from build123d import *

# Parameters (mm, degrees)
SKETCH1_W                   = 50.8
SKETCH1_H                   = 31.75
BASE_LEG_DEPTH              = 4.7625
SKETCH2_W                   = 50.8
SKETCH2_H                   = 31.75
PERPENDICULAR_LEG_DEPTH     = 4.7625
FILLET1_R                   = 2.032
F_32_0_116_DIAMETER_HOLE1_D = 2.9464
W_0_386_DIAMETER_HOLE1_D    = 9.8044
SKETCH15_W                  = 6.549717957
SKETCH15_H                  = 10.713777056
CUT_EXTRUDE2_DEPTH          = 3.81


with BuildPart() as part:
    # Sketch1 → Base leg (new body)
    with BuildSketch(Plane(origin=(0, 0, 0), x_dir=(1, 0, 0), z_dir=(0, 1, 0))):
        with Locations((25.4, -15.875)):
            Rectangle(SKETCH1_W, SKETCH1_H)
    extrude(amount=BASE_LEG_DEPTH)

    # Sketch2 → Perpendicular leg (add)
    with BuildSketch(Plane.XY):
        with Locations((25.4, 15.875)):
            Rectangle(SKETCH2_W, SKETCH2_H)
    extrude(amount=PERPENDICULAR_LEG_DEPTH)

    # Fillet1
    fillet1_edges = [part.edges().sort_by_distance(p)[0] for p in [
        (25.4, 31.75, 4.7625),
        (25.4, 4.7625, 31.75),
    ]]
    fillet(fillet1_edges, radius=FILLET1_R)

    # #32 (0.116) Diameter Hole1 (through all)
    with Locations(Plane(origin=(0, 0, 0), x_dir=(-1, 0, 0), z_dir=(0, -1, 0))):
        with Locations((-38.1, -19.05), (-12.7, -19.05)):
            Hole(F_32_0_116_DIAMETER_HOLE1_D / 2)

    # W (0.386) Diameter Hole1 (through all)
    with Locations(Plane(origin=(0, 0, 0), x_dir=(-1, 0, 0), z_dir=(0, 0, -1))):
        with Locations((-12.7, 19.05), (-38.1, 19.05)):
            Hole(W_0_386_DIAMETER_HOLE1_D / 2)

    # Sketch15 → Cut-Extrude2 (cut)
    with BuildSketch(Plane(origin=(0, 4.7625, 0), x_dir=(1, 0, 0), z_dir=(0, 1, 0))):
        with Locations((2.926349869, -25.756092966)):
            Rectangle(SKETCH15_W, SKETCH15_H)
    extrude(amount=-CUT_EXTRUDE2_DEPTH, mode=Mode.SUBTRACT)


solid = part.part
Input: part model. Units: mm. Frame: model coordinates. A direction names the side the tool comes from. Coordinates: 2 decimals unless noted, no trailing zeros. Loops run counter-clockwise (first coordinate to the right, second up) from the corner with the lowest first, then second, coordinate; pieces in that order, holes last. Notation, with made-up numbers: (84, -35) - (111, -35) arc R20 cw to (111, -30) - close; hole circle Ø1 at (80, -39.75). An arc over 180 degrees is marked (long way). Answer in a Markdown table with one row per item. Add a question column.
Item 1: Access query for faces 5 (the flat face through (0, 10, 4)), 6 (the flat face through (3, 3, 20.399)), 7 (the flat face through (25, 4.762, 17)). Directions: +Z, -Z, +X, -X, +Y, -Y. A direction counts if a zero-diameter tool reaches every point of the face in a straight line with its end or side. Return the directions, or none.
Item 2: Mould query, pull axis Z, two halves, no side actions, for faces 1 (the flat face through (6.201, 3, 26)), 2 (the flat face through (25, 16, 0)), 3 (the cylindrical face through (42.776, 20.522, 2.415)), 4 (the flat face through (25, 1, 31.75)). Classes: released by +Z, released by -Z, zero draft, split by the parting line, or undercut.
Item 3: Section query A-A on y = 19.05. Return the cut outline in (x, z).
Item 4: Contact query for flat-ended pins moving along their axis: P1, Ø5, axis at x = 10.5, z = 26, coming from the +Y side; P2, Ø5, axis at y = 8.5, z = 16, coming from the -X side; P3, Ø12.5, axis at x = 21.5, y = 22, coming from the +Z side; P4, Ø4, axis at x = 26, y = 19.5, coming from the -Z side. Output: stop coordinate, or through.
Item 5: Section query C-C on z = 19.05. Return the cut outline in (x, y).
Item 6: Section query D-D on y = 13.5. Return the cut outline in (x, z), then the cut area to 3 significant figures.
Item 7: Section query B-B on x = 12.7. Return the cut outline in (y, z).
Item 8: Line query: line 1 along X through (y, z) = (1.2, 19.05); line 2 along X through (y, z) = (19, 2); line 3 along Z through (x, y) = (38, 2). Output: solid intervals per line, ascending. Write a range as [from, to].
Recorded:
| question | item | result |
|---|---|---|
| 1 | face 5 | +Z, -Z, -X, +Y, -Y |
| 1 | face 6 | -X, +Y |
| 1 | face 7 | +Z, +X, -X, +Y |
| 2 | face 1 | undercut |
| 2 | face 2 | released by -Z |
| 2 | face 3 | zero draft |
| 2 | face 4 | released by +Z |
| 3 | outline | (0, 0) - (7.8, 0) - (7.8, 4.76) - (0, 4.76) - close; (17.6, 0) - (33.2, 0) - (33.2, 4.76) - (17.6, 4.76) - close; (43, 0) - (50.8, 0) - (50.8, 4.76) - (43, 4.76) - close |
| 4 | P1 | y = 4.76 |
| 4 | P2 | through |
| 4 | P3 | z = 4.76 |
| 4 | P4 | z = 0 |
| 5 | outline | (0, 0) - (11.23, 0) - (11.23, 4.76) - (0, 4.76) - close; (14.17, 0) - (36.63, 0) - (36.63, 4.76) - (14.17, 4.76) - close; (39.57, 0) - (50.8, 0) - (50.8, 4.76) - (39.57, 4.76) - close |
| 6 | outline | (0, 0) - (50.8, 0) - (50.8, 4.76) - (0, 4.76) - close |
| 6 | area | 242 mm^2 |
| 7 | outline | (0, 0) - (14.15, 0) - (14.15, 4.76) - (4.76, 4.76) - (4.76, 17.58) - (0, 17.58) - close; (0, 20.52) - (4.76, 20.52) - (4.76, 29.72) arc R2.03 ccw to (2.73, 31.75) - (0, 31.75) - close; (23.95, 0) - (31.75, 0) - (31.75, 2.73) arc R2.03 ccw to (29.72, 4.76) - (23.95, 4.76) - close |
| 8 | line 1 | [0, 11.23], [14.17, 36.63], [39.57, 50.8] |
| 8 | line 2 | [0, 7.8], [17.6, 33.2], [43, 50.8] |
| 8 | line 3 | [0, 17.58], [20.52, 31.75] |
